Build history of the part. All positions in model axes, mm. Round coordinates to 2 decimals unless told otherwise and drop trailing zeros. Loops run counter-clockwise (first coordinate to the right, second up) from the corner with the lowest first, then second, coordinate; pieces in that order, holes last. Notation, with made-up numbers: (64.5, 48) -> (89.5, 48) arc R15 ccw to (89.5, 54) -> close; hole circle Ø4 at (-14, 44). An arc over 180 degrees is marked (long way). Put each result on its own line as item: value. Start each with the question number.
Item 1: Cut at A-A, the plane y = -2.5. List the corners of the cut face in (x, z).
Item 2: Cut at C-C, the plane z = -5.5. List the corners of the cut face in (x, y).
Item 3: Flat gauge pins, fed straight in: pin 1 Ø3 at (y, z) = (-2.5, 10.5) entering from -X; pin 2 Ø3 at (x, y) = (58.5, -3) entering from +Z. Where does each tip first touch, or does it go through?
Item 4: Drill centre lines: probe 1 along Z at (x, y) = (-37, -5.25); probe 2 along X at (y, z) = (-3.75, 11); probe 3 along Z at (x, y) = (41, -4.75). Where is each one in solid material? Low to high. Write a range as [from, to].
Item 5: Cut at B-B, the plane x = -37.5. List the corners of the cut face in (y, z).
```python
from build123d import *

# Parameters (mm, degrees)
F0_W     = 69.857972
F0_H     = 25.4
F1_DEPTH = 6.35
F2_W     = 15.100554
F2_H     = 10.679496
F2_W_2   = 114.3
F2_H_2   = 18.241366
F3_DEPTH = 6.35


with BuildPart() as f1:
    # F0 (on Front) → F1 (new body)
    with BuildSketch(Plane.XZ):
        Rectangle(F0_W, F0_H)
    extrude(amount=F1_DEPTH)

    # F2 (on Front) → F3 (join)
    with BuildSketch(Plane.XZ):
        with Locations((-42.164538, 1.567621)):
            Rectangle(F2_W, F2_H)
        with Locations((44.382397, 0)):
            Rectangle(F2_W_2, F2_H_2)
    extrude(amount=F3_DEPTH)


solid = f1.part
```
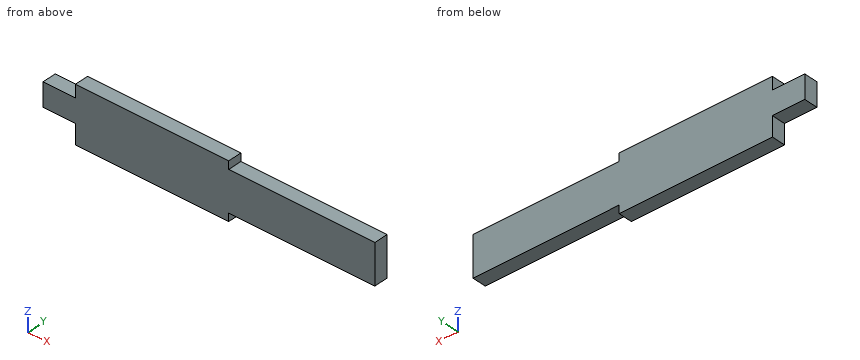
Reply:
1. outline: (-49.71, -3.77) -> (-34.93, -3.77) -> (-34.93, -12.7) -> (34.93, -12.7) -> (34.93, -9.12) -> (101.53, -9.12) -> (101.53, 9.12) -> (34.93, 9.12) -> (34.93, 12.7) -> (-34.93, 12.7) -> (-34.93, 6.91) -> (-49.71, 6.91) -> close
2. outline: (-34.93, -6.35) -> (101.53, -6.35) -> (101.53, 0) -> (-34.93, 0) -> close
3. pin 1: stops at x = -34.93
3. pin 2: stops at z = 9.12
4. probe 1: z = [-3.77, 6.91]
4. probe 2: x = [-34.93, 34.93]
4. probe 3: z = [-9.12, 9.12]
5. outline: (-6.35, -3.77) -> (0, -3.77) -> (0, 6.91) -> (-6.35, 6.91) -> close
